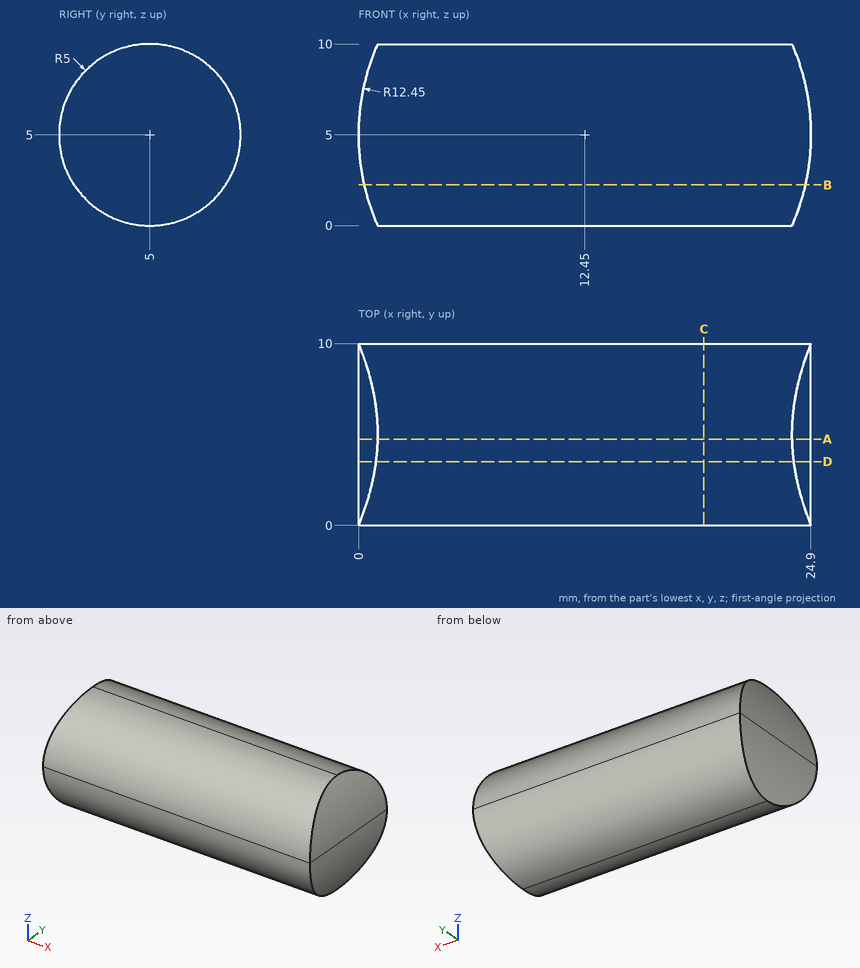
Design review of the part shown in the three views and the two pictorial views. Dimensions are in mm from the part's minimum x, y and z. Give positions to 0.01 mm unless a question says otherwise; leave off trailing zeros. Write each loop counter-clockwise with the first axis right and the second up, starting at its lowest first coordinate (ties: lowest second). Pieces come first, ordered by that corner, then holes.
(1) Add section C-C (x = 19). Give the boundary of the cut face in (y, z), and give its area (3 significant figures).
Checked values:
outline: circle Ø10 at (5, 5)
area: 78.5 mm2
(2) Wall thickness on line 1 along Z through (x, y) = (20.5, 5.25); line 2 along Y through (x, z) = (7.25, 9); line 3 along Y through (x, z) = (21, 6.75): over which ranges is each line inside the solid? List them lowest first.
Checked values:
line 1: z = 0.01 to 9.99
line 2: y = 2 to 8
line 3: y = 0.32 to 9.68
(3) Clearance check with flat-ended pins moving along their axes: pin 1 Ø1.5 at (x, y) = (15.5, 3) entering from +Z; pin 2 Ø3 at (x, z) = (21.5, 3) entering from -Y. State where each tip first meets the part, or that it passes through.
Checked values:
pin 1: stops at z = 9.84
pin 2: stops at y = 0.03
(4) Add section A-A (y = 4.75). Give the boundary of the cut face in (x, z), and give its area (3 significant figures).
Checked values:
outline: (1.05, 0.01) - (23.85, 0.01) arc R12.45 ccw to (23.85, 9.99) - (1.05, 9.99) arc R12.45 ccw to start
area: 242 mm2
(5) Add section B-B (z = 2.25). Give the boundary of the cut face in (x, y), and give its area (3 significant figures).
Checked values:
outline: (0.31, 0.82) - (24.59, 0.82) - (24.59, 9.18) - (0.31, 9.18) - close
area: 203 mm2
(6) Add section D-D (y = 3.5). Give the boundary of the cut face in (x, z).
Checked values:
outline: (0.95, 0.23) - (23.95, 0.23) arc R12.45 ccw to (23.95, 9.77) - (0.95, 9.77) arc R12.45 ccw to start
